```python
from build123d import *

# Parameters (mm, degrees)
F1_DEPTH = 18
F2_R     = 5
F3_R     = 2
F4_R     = 2


with BuildPart() as f1:
    # F0 (on Top) → F1 (new body)
    with BuildSketch(Plane.XY):
        with BuildLine():
            Line((42.340133, 55.661296), (-38.659867, 55.661296))
            ThreePointArc((-38.659867, 55.661296), (-60.580177, 46.581606), (-69.659867, 24.661296))
            ThreePointArc((-69.659867, 24.661296), (-49.931318, -4.216973), (-15.856358, 3.661296))
            Line((-15.856358, 3.661296), (1.840133, 3.661296))
            Line((1.840133, 3.661296), (19.536625, 3.661296))
            ThreePointArc((19.536625, 3.661296), (53.611585, -4.216973), (73.340133, 24.661296))
            ThreePointArc((73.340133, 24.661296), (64.260443, 46.581606), (42.340133, 55.661296))
        make_face()
    extrude(amount=F1_DEPTH)

    # F2
    f2_edges = [f1.edges().sort_by_distance(p)[0] for p in [
        (19.536625, 3.661296, 9),
        (-15.856358, 3.661296, 9),
    ]]
    fillet(f2_edges, radius=F2_R)

    # F3
    f3_edges = [f1.edges().sort_by_distance(p)[0] for p in [
        (71.106916, 13.108278, 18),
        (19.303724, 3.301099, 18),
        (1.840133, 55.661296, 18),
        (1.840133, 3.661296, 18),
        (-67.426649, 13.108278, 18),
        (-15.623458, 3.301099, 18),
    ]]
    fillet(f3_edges, radius=F3_R)

    # F4
    f4_edges = [f1.edges().sort_by_distance(p)[0] for p in [
        (-67.426649, 13.108278, 0),
        (-15.623458, 3.301099, 0),
        (1.840133, 55.661296, 0),
        (1.840133, 3.661296, 0),
        (71.106916, 13.108278, 0),
        (19.303724, 3.301099, 0),
    ]]
    fillet(f4_edges, radius=F4_R)


solid = f1.part
```
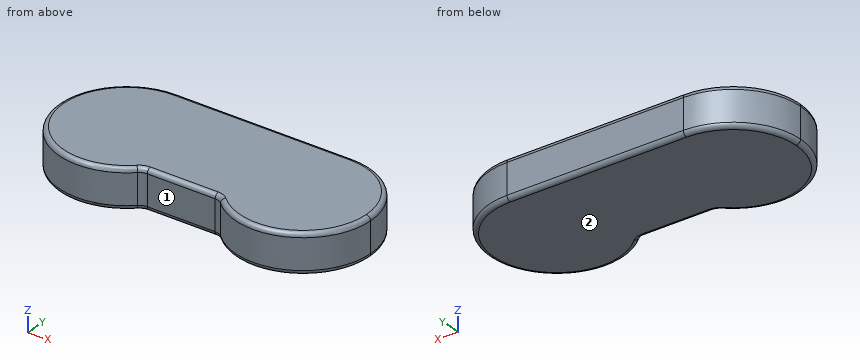
The listing builds one solid part. Answer for the finished solid, in the listing's coordinates (mm). Face numbers are marked on the shaded views. Coordinates: 2 decimals unless noted, no trailing zeros. Write each loop counter-clockwise with the first axis right and the second up, starting at its lowest first coordinate (ties: lowest second). Pieces come first, ordered by that corner, then holes. Notation, with made-up numbers: (33.5, 47.25) - (54.5, 47.25) arc R5 cw to (54.5, 56.25) - close; hole circle Ø9 at (56.5, 81). An arc over 180 degrees is marked (long way). One line per item, written item: value.
1) Find section B-B (x = -5). Give the vertices of the cut face in (y, z), and give its area (3 significant figures).
Geometry check:
outline: (3.66, 2) arc R2 ccw to (5.66, 0) - (53.66, 0) arc R2 ccw to (55.66, 2) - (55.66, 16) arc R2 ccw to (53.66, 18) - (5.66, 18) arc R2 ccw to (3.66, 16) - close
area: 933 mm2
2) For a pull along X with two mould halves and no side action, classify the marked faces 1 and 2 as pulls with the +X half, pulls with the -X half, needs draft (parallel to the pull), parting line crosses it, or undercut.
Geometry check:
face 1: undercut
face 2: needs draft
3) Consider line 1 along Y through (x, z) = (41, 13); line 2 along Y through (x, z) = (-40, 6.5); line 3 along X through (y, z) = (0.5, 7). Determine where each line is inside the solid, lowest interval first. Write a range as from..to.
Geometry check:
line 1: y = -6.31..55.66
line 2: y = -6.31..55.63
line 3: x = -58.08..-19.24, 22.92..61.76
4) Find section A-A (z = 9.75). Give the vertices of the cut face in (x, y), and give its area (3 significant figures).
Geometry check:
outline: (-38.66, 55.66) arc R31 ccw (long way) to (-17.22, 2.27) arc R5 cw to (-13.76, 3.66) - (17.44, 3.66) arc R5 cw to (20.9, 2.27) arc R31 ccw to (73.34, 24.66) arc R31 ccw to (42.34, 55.66) - close
area: 7,550 mm2
5) Each of these flat-tipped pins is pushed along its axis until it touches: pin 1 Ø1.5 at (x, z) = (-15.5, 6) entering from -Y; pin 2 Ø5 at (x, z) = (-45, 6.5) entering from +Y; pin 3 Ø4 at (y, z) = (20.5, 11.5) entering from -X. Where does it stop, or does it pass through?
Geometry check:
pin 1: stops at y = 3
pin 2: stops at y = 55.42
pin 3: stops at x = -69.58
